Geometry: final body of the model. Coordinates: model frame, mm. A direction names the side the tool comes from. Round coordinates to 2 decimals unless told otherwise and drop trailing zeros. Loops run counter-clockwise (first coordinate to the right, second up) from the corner with the lowest first, then second, coordinate; pieces in that order, holes last. Notation, with made-up numbers: (-11.75, 22) - (-3.75, 22) arc R26 ccw to (-3.75, 39) - close; hole circle Ø4 at (-16, 69.5). An arc over 180 degrees is marked (long way). Write item = value, one per line. Start each with the question number.
Item 1: Line query: line 1 (Y direction, x = 4, z = 0.8); line 2 (X direction, y = -23, z = 0.45); line 3 (X direction, y = -15.5, z = 0.9). Output: solid intervals per line, ascending. Write a range as from..to.
Item 2: Access query for faces 1 (the flat face through (0, 30.5, 1)), 2 (the flat face through (-9.5, 0, 1)). Directions: +Z, -Z, +X, -X, +Y, -Y. A direction counts if a zero-diameter tool reaches every point of the face in a straight line with its end or side. Return the directions, or none.
Item 3: Section D-D (y = 25). Return loops of the section in (x, z), plus the area to 3 significant figures.
Item 4: First-contact query: pin 1 (12 mm diameter, centred on x = 8, y = 20.5, fed in from -Z); pin 2 (0.8 mm diameter, centred on y = -1.5, z = 1, fed in from +X); pin 3 (0.8 mm diameter, centred on y = 4, z = 1, fed in from -X). Flat tips, straight axial feed; report the tip coordinate or a pass-through.
Item 5: Section C-C (z = 1). Count the separate pieces of the cut face and the enclosed holes in it, plus the area to 3 significant figures.
Item 6: Section B-B (y = 16). Return loops of the section in (x, z).
Item 7: Draft query along Y for faces 3 (the cylindrical face through (-10.878, 29.847, 0.764)), 4 (the cylindrical face through (-22.06, -23.91, 0.76)), 5 (the cylindrical face through (-10.741, -29.882, 0.764)). Return one class per face: pulls with the +Y half, pulls with the -Y half, needs draft (parallel to the pull), parting line crosses it, or undercut.
Item 8: Section A-A (x = -0.5). Return loops of the section in (y, z), plus the area to 4 significant figures.
from build123d import *

# Parameters (mm, degrees)
ESQUISSE1_R             = 1.65
BOSS_EXTRU_1_DEPTH      = 1.55
ESQUISSE2_W             = 19
ESQUISSE2_H             = 42
ENL_V_MAT_EXTRU_1_DEPTH = 46.281370341
CONG_1_R                = 10
CONG_2_R                = 1
ESQUISSE3_OUTSIDE_W     = 84.104
ESQUISSE3_OUTSIDE_H     = 84.104
ESQUISSE3_OUTSIDE_W_2   = 70
ESQUISSE3_OUTSIDE_H_2   = 61
ENL_V_MAT_EXTRU_2_DEPTH = 46.281370486
CONG_3_R                = 20


with BuildPart() as part:
    # Esquisse1 → Boss.-Extru.1 (new body)
    with BuildSketch(Plane.XY):
        with BuildLine():
            ThreePointArc((-24.957906965, 20.02755302), (-32, 0), (-24.957906965, -20.02755302))
            ThreePointArc((-24.957906965, -20.02755302), (-24.748737342, -24.748737342), (-20.02755302, -24.957906965))
            ThreePointArc((-20.02755302, -24.957906965), (0, -32), (20.02755302, -24.957906965))
            ThreePointArc((20.02755302, -24.957906965), (24.748737342, -24.748737342), (24.957906965, -20.02755302))
            ThreePointArc((24.957906965, -20.02755302), (32, 0), (24.957906965, 20.02755302))
            ThreePointArc((24.957906965, 20.02755302), (24.748737342, 24.748737342), (20.02755302, 24.957906965))
            ThreePointArc((20.02755302, 24.957906965), (0, 32), (-20.02755302, 24.957906965))
            ThreePointArc((-20.02755302, 24.957906965), (-24.748737342, 24.748737342), (-24.957906965, 20.02755302))
        make_face()
        with Locations(Location((-22.273863607, 22.273863607, 0), (0, 0, 180))):
            Circle(ESQUISSE1_R, mode=Mode.SUBTRACT)
        with Locations(Location((22.273863607, 22.273863607, 0), (0, 0, 180))):
            Circle(ESQUISSE1_R, mode=Mode.SUBTRACT)
        with Locations(Location((22.273863607, -22.273863607, 0), (0, 0, 180))):
            Circle(ESQUISSE1_R, mode=Mode.SUBTRACT)
        with Locations(Location((-22.273863607, -22.273863607, 0), (0, 0, 180))):
            Circle(ESQUISSE1_R, mode=Mode.SUBTRACT)
    extrude(amount=BOSS_EXTRU_1_DEPTH)

    # Esquisse2 → Enlèv. mat.-Extru.1 (cut, through all)
    with BuildSketch(Plane.XY.offset(1.55)):
        Rectangle(ESQUISSE2_W, ESQUISSE2_H)
    extrude(amount=-ENL_V_MAT_EXTRU_1_DEPTH, mode=Mode.SUBTRACT)

    # Congé1
    cong_1_edges = [part.edges().sort_by_distance(p)[0] for p in [
        (20.02755302, 24.957906965, 0.775),
        (24.957906965, 20.02755302, 0.775),
        (24.957906965, -20.02755302, 0.775),
        (20.02755302, -24.957906965, 0.775),
        (-20.02755302, -24.957906965, 0.775),
        (-24.957906965, -20.02755302, 0.775),
        (-24.957906965, 20.02755302, 0.775),
        (-20.02755302, 24.957906965, 0.775),
    ]]
    fillet(cong_1_edges, radius=CONG_1_R)

    # Congé2
    cong_2_edges = [part.edges().sort_by_distance(p)[0] for p in [
        (-9.5, -21, 0.775),
        (-9.5, 21, 0.775),
        (9.5, 21, 0.775),
        (9.5, -21, 0.775),
    ]]
    fillet(cong_2_edges, radius=CONG_2_R)

    # Esquisse3 outside → Enlèv. mat.-Extru.2 (cut, through all)
    with BuildSketch(Plane.XY.offset(1.55)):
        Rectangle(ESQUISSE3_OUTSIDE_W, ESQUISSE3_OUTSIDE_H)
        Rectangle(ESQUISSE3_OUTSIDE_W_2, ESQUISSE3_OUTSIDE_H_2, mode=Mode.SUBTRACT)
    extrude(amount=-ENL_V_MAT_EXTRU_2_DEPTH, mode=Mode.SUBTRACT)

    # Congé3
    cong_3_edges = [part.edges().sort_by_distance(p)[0] for p in [
        (9.682458366, -30.5, 0.775),
        (-9.682458366, -30.5, 0.775),
        (-9.682458366, 30.5, 0.775),
        (9.682458366, 30.5, 0.775),
    ]]
    fillet(cong_3_edges, radius=CONG_3_R)


solid = part.part
Taken from the geometry:
q1.line_1 = -30.5..-21, 21..30.5
q1.line_2 = -25.7..-23.76, -20.79..20.79, 23.76..25.7
q1.line_3 = -28..-9.5, 9.5..28
q2.face_1 = +Z, -Z, +X, -X, +Y
q2.face_2 = +Z, -Z
q3.outline = (-24.47, 0) - (24.47, 0) - (24.47, 1.55) - (-24.47, 1.55) - close
q3.area = 75.9 mm^2
q4.pin_1 = 0
q4.pin_2 = 31.98
q4.pin_3 = -31.8
q5.separate_pieces = 1
q5.enclosed_holes = 5
q5.area = 2,420 mm^2
q6.outline = (-27.71, 0) - (-9.5, 0) - (-9.5, 1.55) - (-27.71, 1.55) - close; (9.5, 0) - (27.71, 0) - (27.71, 1.55) - (9.5, 1.55) - close
q7.face_3 = pulls with the +Y half
q7.face_4 = undercut
q7.face_5 = pulls with the -Y half
q8.outline = (-30.5, 0) - (-21, 0) - (-21, 1.55) - (-30.5, 1.55) - close; (21, 0) - (30.5, 0) - (30.5, 1.55) - (21, 1.55) - close
q8.area = 29.45 mm^2
